```python
from build123d import *

# Parameters (mm, degrees)
F0_W     = 50
F0_H     = 70
F1_DEPTH = 3
F4_D     = 3
F8_DEPTH = 28.640468
F9_R     = 10


with BuildPart() as f1:
    # F0 (on Top) → F1 (new body)
    with BuildSketch(Plane.XY):
        with Locations((25, 35)):
            Rectangle(F0_W, F0_H)
    extrude(amount=F1_DEPTH)

    # F4 (through all)
    with Locations(Plane.XY.offset(3)):
        with Locations((10, 25), (10, 50)):
            Hole(F4_D / 2)

    # F7 (on face) → F8 (cut)
    with BuildSketch(Plane.XY.offset(3)):
        with BuildLine():
            ThreePointArc((35, 15), (37.5, 12.5), (40, 15))
            Line((40, 15), (40, 55))
            ThreePointArc((40, 55), (37.5, 57.5), (35, 55))
            Line((35, 55), (35, 15))
        make_face()
    extrude(amount=-F8_DEPTH, mode=Mode.SUBTRACT)

    # F9
    f9_edges = [f1.edges().sort_by_distance(p)[0] for p in [
        (50, 70, 1.5),
        (50, 0, 1.5),
    ]]
    fillet(f9_edges, radius=F9_R)

    # F10: F1 across plane


with BuildPart() as f1_1:
    add(f1.part)
    add(f1.part.mirror(Plane.YZ))


solid = f1_1.part
```
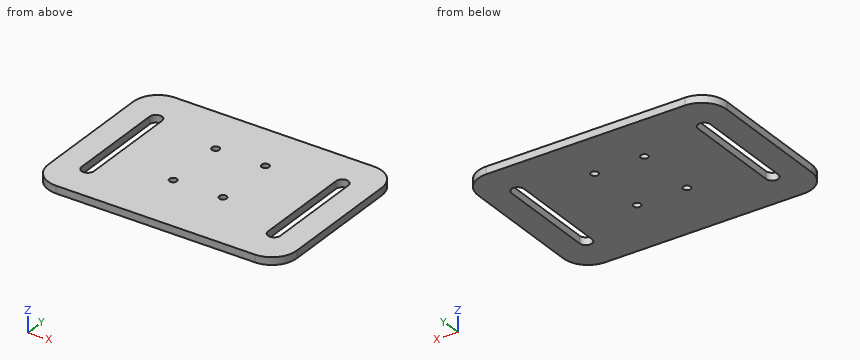
Model file for the job. Use its own axes, mm. Coordinates: 2 decimals unless noted, no trailing zeros. Order: outer loops, then holes, each group sorted by start corner. A loop starts at its lowest first (then second) coordinate and runs counter-clockwise, first axis right, second up. Notation, with made-up numbers: (-13.5, -13.5) -> (41.5, -13.5) arc R36 ccw to (41.5, 23.5) -> close; hole circle Ø4 at (14, 36). An arc over 180 degrees is marked (long way). Answer as a JSON object with one key per item and string values. Group by question number.
1) Cut at D-D, the plane x = -37.5. Write the cut outline in (y, z), then the cut area to 3 significant figures.
2) Cut at C-C, the plane z = 1.5. Write the cut outline in (x, y).
3) Drill centre lines: L1, parallel to Y at x = 10, z = 0.85; L2, parallel to X at y = 53, z = 0.7; L3, parallel to X at y = 26, z = 2.85. Where is each one in solid material? Low to high.
4) Cut at A-A, the plane x = -10. Write the cut outline in (y, z).
5) Cut at B-B, the plane y = 50. Write the cut outline in (x, z).
Check values:
{
 "1": {"outline": "(0, 0) -> (12.5, 0) -> (12.5, 3) -> (0, 3) -> close; (57.5, 0) -> (70, 0) -> (70, 3) -> (57.5, 3) -> close", "area": "75.0 mm²"},
 "2": {"outline": "(-50, 10) arc R10 ccw to (-40, 0) -> (40, 0) arc R10 ccw to (50, 10) -> (50, 60) arc R10 ccw to (40, 70) -> (-40, 70) arc R10 ccw to (-50, 60) -> close; hole (-40, 15) arc R2.5 ccw to (-35, 15) -> (-35, 55) arc R2.5 ccw to (-40, 55) -> close; hole circle Ø3 at (-10, 25); hole circle Ø3 at (-10, 50); hole circle Ø3 at (10, 25); hole circle Ø3 at (10, 50); hole (35, 15) arc R2.5 ccw to (40, 15) -> (40, 55) arc R2.5 ccw to (35, 55) -> close"},
 "3": {"L1": "y = 0 to 23.5, 26.5 to 48.5, 51.5 to 70", "L2": "x = -50 to -40, -35 to 35, 40 to 50", "L3": "x = -50 to -40, -35 to -11.12, -8.88 to 8.88, 11.12 to 35, 40 to 50"},
 "4": {"outline": "(0, 0) -> (23.5, 0) -> (23.5, 3) -> (0, 3) -> close; (26.5, 0) -> (48.5, 0) -> (48.5, 3) -> (26.5, 3) -> close; (51.5, 0) -> (70, 0) -> (70, 3) -> (51.5, 3) -> close"},
 "5": {"outline": "(-50, 0) -> (-40, 0) -> (-40, 3) -> (-50, 3) -> close; (-35, 0) -> (-11.5, 0) -> (-11.5, 3) -> (-35, 3) -> close; (-8.5, 0) -> (8.5, 0) -> (8.5, 3) -> (-8.5, 3) -> close; (11.5, 0) -> (35, 0) -> (35, 3) -> (11.5, 3) -> close; (40, 0) -> (50, 0) -> (50, 3) -> (40, 3) -> close"}
}
